Source: CAD feature listing. Evaluate the final solid. Frame: model axes, mm. Face numbers are marked on the shaded views. Give positions to 0.01 mm unless a question says otherwise; leave off trailing zeros. Write each loop counter-clockwise with the first axis right and the second up, starting at its lowest first coordinate (ties: lowest second). Pieces come first, ordered by that corner, then holes. Notation, with made-up numbers: (53, 8) - (72, 8) arc R12 cw to (72, 28) - close; hole circle Ø6 at (72.5, 21). An arc over 180 degrees is marked (long way). Answer as a JSON object with one key per item and string values. Group by question number.
from build123d import *

# Parameters (mm, degrees)
ESTRUSIONE_ESTRUSIONE1_DEPTH = 2
SCHIZZO3_R                   = 4.5
TAGLIO_ESTRUSIONE1_DEPTH     = 2


with BuildPart() as part:
    # Schizzo2 → Estrusione-Estrusione1 (new body)
    with BuildSketch(Plane.XY):
        with BuildLine():
            Line((-21, 2.5), (-21, -2.5))
            Line((-21, -2.5), (-6, -2.5))
            ThreePointArc((-6, -2.5), (-6.5, 0), (-6, 2.5))
            Line((-6, 2.5), (-21, 2.5))
        make_face()
        with BuildLine():
            ThreePointArc((-6, 2.5), (-6.5, 0), (-6, -2.5))
            Line((-6, -2.5), (6, -2.5))
            ThreePointArc((6, -2.5), (6.373774392, -1.274754878), (6.5, 0))
            ThreePointArc((6.5, 0), (6.373774392, 1.274754878), (6, 2.5))
            Line((6, 2.5), (-6, 2.5))
        make_face()
        with BuildLine():
            ThreePointArc((6.5, 0), (6.373774392, -1.274754878), (6, -2.5))
            Line((6, -2.5), (21, -2.5))
            Line((21, -2.5), (21, 2.5))
            Line((21, 2.5), (6, 2.5))
            ThreePointArc((6, 2.5), (6.373774392, 1.274754878), (6.5, 0))
        make_face()
        with BuildLine():
            ThreePointArc((6, 2.5), (0, 6.5), (-6, 2.5))
            Line((-6, 2.5), (6, 2.5))
        make_face()
        with BuildLine():
            Line((6, -2.5), (-6, -2.5))
            ThreePointArc((-6, -2.5), (0, -6.5), (6, -2.5))
        make_face()
    extrude(amount=ESTRUSIONE_ESTRUSIONE1_DEPTH)

    # Schizzo3 → Taglio-Estrusione1 (cut)
    with BuildSketch(Plane.XY.offset(2)):
        Circle(SCHIZZO3_R)
    extrude(amount=-TAGLIO_ESTRUSIONE1_DEPTH, mode=Mode.SUBTRACT)


solid = part.part
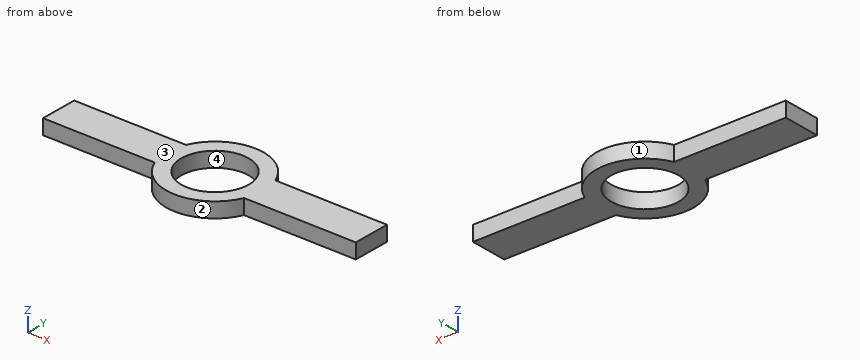
Q1. Section D-D on x = 11. Return the cut outline in (y, z), then the cut area to 3 significant figures.
Q2. Section C-C on z = 1.5. Return the cut outline in (x, y).
Q3. Ray query, probe 1 along Y at (x, z) = (0, 1.6); probe 2 along Y at (x, z) = (9, 0.15); probe 3 along Y at (x, z) = (2.5, 1.4). Return the intervals inside material, ascending. Write a range as [from, to].
Q4. First-contact query: pin 1 Ø1 at (x, z) = (-15, 1) entering from +Y; pin 2 Ø1 at (x, z) = (16.5, 0.5) entering from -Y. Flat tips, straight axial feed; report the tip coordinate or a pass-through.
Q5. Section A-A on y = 0. Return the cut outline in (x, z), then the cut area to 3 significant figures.
Q6. Draft query along Y for the marked faces 1, 2, 3 and 4. Return one class per face: released by +Y, released by -Y, zero draft, split by the parting line, or undercut.
Q7. Section B-B on x = 0. Return the cut outline in (y, z).
Taken from the geometry:
{
 "1": {"outline": "(-2.5, 0) - (2.5, 0) - (2.5, 2) - (-2.5, 2) - close", "area": "10.0 mm²"},
 "2": {"outline": "(-21, -2.5) - (-6, -2.5) arc R6.5 ccw to (6, -2.5) - (21, -2.5) - (21, 2.5) - (6, 2.5) arc R6.5 ccw to (-6, 2.5) - (-21, 2.5) - close; hole circle Ø9 at (0, 0)"},
 "3": {"probe 1": "y = [-6.5, -4.5], [4.5, 6.5]", "probe 2": "y = [-2.5, 2.5]", "probe 3": "y = [-6, -3.74], [3.74, 6]"},
 "4": {"pin 1": "stops at y = 2.5", "pin 2": "stops at y = -2.5"},
 "5": {"outline": "(-21, 0) - (-4.5, 0) - (-4.5, 2) - (-21, 2) - close; (4.5, 0) - (21, 0) - (21, 2) - (4.5, 2) - close", "area": "66.0 mm²"},
 "6": {"face 1": "released by +Y", "face 2": "released by -Y", "face 3": "zero draft", "face 4": "undercut"},
 "7": {"outline": "(-6.5, 0) - (-4.5, 0) - (-4.5, 2) - (-6.5, 2) - close; (4.5, 0) - (6.5, 0) - (6.5, 2) - (4.5, 2) - close"}
}
